```python
from build123d import *

# Parameters (mm, degrees)
F0_R     = 9.5
F1_DEPTH = 100
F2_R     = 12.7
F2_R_2   = 9.5
F3_DEPTH = 25
F4_R     = 6.35
F5_DEPTH = 37.5
F4_R_2   = 4
F6_DEPTH = 12.5
F7_SIZE  = 2.5
F8_SIZE  = 1


with BuildPart() as f1:
    # F0 (on Right) → F1 (new body, symmetric)
    with BuildSketch(Plane.YZ):
        Circle(F0_R)
    extrude(amount=F1_DEPTH, both=True)

    # F2 (on face) → F3 (join)
    with BuildSketch(Plane.YZ.offset(100)):
        Circle(F2_R)
        Circle(F2_R_2, mode=Mode.SUBTRACT)
    extrude(amount=-F3_DEPTH)

    # F4 (on Top) → F5 (join, symmetric)
    with BuildSketch(Plane.XY):
        with Locations((87.7, 0)):
            Circle(F4_R)
    extrude(amount=F5_DEPTH, both=True)

    # F4 (on Top) → F6 (cut, symmetric)
    with BuildSketch(Plane.XY):
        with Locations((-90, 0)):
            Circle(F4_R_2)
    extrude(amount=F6_DEPTH, both=True, mode=Mode.SUBTRACT)

    # F7
    f7_edges = [f1.edges().sort_by_distance(p)[0] for p in [
        (-100, -9.5, 0),
    ]]
    chamfer(f7_edges, length=F7_SIZE)

    # F8
    f8_edges = [f1.edges().sort_by_distance(p)[0] for p in [
        (75, -12.7, 0),
        (100, -12.7, 0),
        (81.35, 0, -37.5),
        (81.35, 0, 37.5),
    ]]
    chamfer(f8_edges, length=F8_SIZE)


solid = f1.part
```
Geometry check sheet. Reference: the model listing, model coordinates, mm. A direction names the side the tool comes from. Coordinates: 2 decimals unless noted, no trailing zeros. Order: outer loops, then holes, each group sorted by start corner. A loop starts at its lowest first (then second) coordinate and runs counter-clockwise, first axis right, second up. Notation, with made-up numbers: (17.25, 42) - (59.25, 42) arc R13 ccw to (59.25, 65) - close; hole circle Ø11 at (-8, 3). An arc over 180 degrees is marked (long way). Answer as a JSON object with one key per item and string values. Group by question number.
Item 1: Depth check by flat-ended pin: pin 1 Ø1.5 at (x, y) = (-7.5, -2) entering from +Z; pin 2 Ø6 at (x, y) = (-5, 2.5) entering from +Z; pin 3 Ø3 at (x, y) = (14.5, 9.5) entering from -Z. Enter the tip coordinate at first touch or a pass-through.
Item 2: Sectioned sample at D-D, the plane x = -90. Record the cut outline in (y, z), and give its area (3 significant figures).
Item 3: Sectioned sample at C-C, the plane x = 87.7. Record the cut outline in (y, z).
Item 4: Tool access check on faces 5 (the face through (-10.043, 8.776, -3.639)), 6 (the face through (100, 0, 0)), 7 (the face through (93.566, -2.432, 23.928)). Record the directions out of +Z, -Z, +X, -X, +Y, -Y that give a thin tool (end or side, any length) a straight path to the whole face; none if there is none.
Item 5: Draft check along X on faces 1 (the face through (88, 0, 37.5)), 2 (the face through (-100, 0, 0)), 3 (the face through (-94, 0, 0)), 4 (the face through (81.356, 0.279, -23.571)). Enter one of: +X half, -X half, draft (parallel to the pull), parting line (faces both ways), or undercut.
Item 6: Scan lines: probe 1 along X at (y, z) = (0, 4.5); probe 2 along X at (y, z) = (4, -9.5); probe 3 along X at (y, z) = (-0.25, -15). Record each from-to range of solid material in increasing order.
Item 7: Sectioned sample at B-B, the plane z = 0. Record the cut outline in (x, y).
Resolved:
{
 "1": {"pin 1": "z = 9.42", "pin 2": "z = 9.5", "pin 3": "z = -5.12"},
 "2": {"outline": "(-4, -8.62) - (-4, 8.62) arc R9.5 ccw to start; (4, -8.62) arc R9.5 ccw to (4, 8.62) - close", "area": "136 mm^2"},
 "3": {"outline": "(-6.35, -36.5) - (-5.35, -37.5) - (5.35, -37.5) - (6.35, -36.5) - (6.35, -11) arc R12.7 ccw to (6.35, 11) - (6.35, 36.5) - (5.35, 37.5) - (-5.35, 37.5) - (-6.35, 36.5) - (-6.35, 11) arc R12.7 ccw to (-6.35, -11) - close"},
 "4": {"face 5": "-X", "face 6": "+Z, -Z, +X, +Y, -Y", "face 7": "+Z"},
 "5": {"face 1": "draft", "face 2": "-X half", "face 3": "undercut", "face 4": "parting line"},
 "6": {"probe 1": "-100 to -94, -86 to 100", "probe 2": "75 to 100", "probe 3": "81.35 to 94.05"},
 "7": {"outline": "(-100, -7) - (-97.5, -9.5) - (75, -9.5) - (75, -11.7) - (76, -12.7) - (99, -12.7) - (100, -11.7) - (100, 11.7) - (99, 12.7) - (76, 12.7) - (75, 11.7) - (75, 9.5) - (-97.5, 9.5) - (-100, 7) - close; hole circle Ø8 at (-90, 0)"}
}
